Build history of the part. All positions in model axes, mm. Face numbers are marked on the shaded views. A direction names the side the tool comes from. Give positions to 0.01 mm unless a question says otherwise; leave off trailing zeros. Order: outer loops, then holes, each group sorted by start corner. A loop starts at its lowest first (then second) coordinate and runs counter-clockwise, first axis right, second up. Notation, with made-up numbers: (5.25, 19) - (29.25, 19) arc R12 cw to (29.25, 42) - close; hole circle Ø6 at (-14, -32). An arc over 180 degrees is marked (long way). Answer in a Markdown table with one row per item.
```python
from build123d import *

# Parameters (mm, degrees)
SKETCH3_R           = 9.525
SKETCH3_R_2         = 3.175
BOSS_EXTRUDE1_DEPTH = 1.905
SKETCH4_R           = 3.175
BOSS_EXTRUDE2_DEPTH = 4.445


with BuildPart() as part:
    # Sketch3 → Boss-Extrude1 (new body)
    with BuildSketch(Plane(origin=(0, 0, 0), x_dir=(1, 0, 0), z_dir=(0, 1, 0))):
        Circle(SKETCH3_R)
        Circle(SKETCH3_R_2, mode=Mode.SUBTRACT)
    extrude(amount=BOSS_EXTRUDE1_DEPTH)

    # Sketch4 → Boss-Extrude2 (add)
    with BuildSketch(Plane(origin=(0, 1.905, 0), x_dir=(1, 0, 0), z_dir=(0, 1, 0))):
        Polygon((6.647647659, 0), (3.323823829, 5.757031748), (-3.323823829, 5.757031748), (-6.647647659, 0), (-3.323823829, -5.757031748), (3.323823829, -5.757031748), align=None)
        Circle(SKETCH4_R, mode=Mode.SUBTRACT)
    extrude(amount=BOSS_EXTRUDE2_DEPTH)


solid = part.part
```
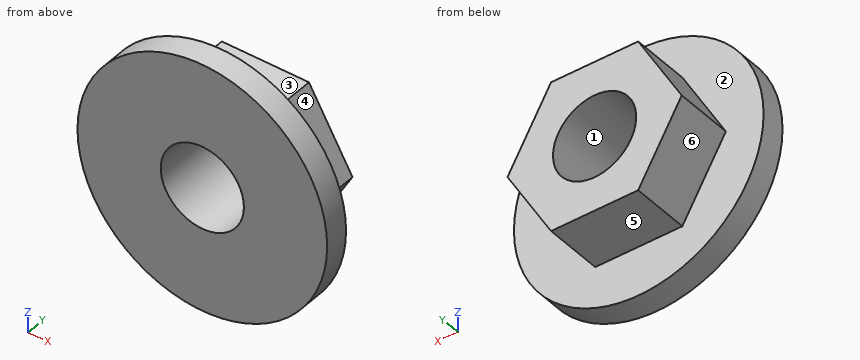
1. Drop flat-ended pins along their axis: P1, Ø1.3, axis at x = -1.5, y = 4, coming from the -Z side; P2, Ø1.3, axis at x = 1, y = 4.5, coming from the +Z side; P3, Ø2, axis at y = 1.5, z = -7.5, coming from the -X side; P4, Ø9.5, axis at x = -0.5, z = 2, coming from the +Y side. Give the stop position or say it passes through.
Check result:
| item | result |
|---|---|
| P1 | stops at z = -5.76 |
| P2 | stops at z = 5.76 |
| P3 | stops at x = -6.96 |
| P4 | stops at y = 6.35 |
2. Cut at D-D on z = -3.5. Write the cut outline in (x, y) (3 decimals).
Check result:
| item | result |
|---|---|
| outline | (-8.859, 0) - (8.859, 0) - (8.859, 1.905) - (4.627, 1.905) - (4.627, 6.35) - (-4.627, 6.35) - (-4.627, 1.905) - (-8.859, 1.905) - close |
3. Which spindle directions (+Z, -Z, +X, -X, +Y, -Y) get a long thin tool onto all of the face, cutting with end or side? Do the marked faces 4, 5 and 6. Say none if no direction does.
Check result:
| item | result |
|---|---|
| face 4 | +Z, +X, +Y |
| face 5 | -Z, +X, -X, +Y |
| face 6 | -Z, -X, +Y |
4. Cut at C-C on x = 6.25. Write the cut outline in (y, z) (3 decimals), and give its area (3 significant figures).
Check result:
| item | result |
|---|---|
| outline | (0, -7.188) - (1.905, -7.188) - (1.905, -0.689) - (6.35, -0.689) - (6.35, 0.689) - (1.905, 0.689) - (1.905, 7.188) - (0, 7.188) - close |
| area | 33.5 mm² |
5. Two-plate mould, pull along Z, no slides. Class the marked faces 1, 2 and 3: +Z half, -Z half, draft (parallel to the pull), parting line (faces both ways), or undercut.
Check result:
| item | result |
|---|---|
| face 1 | undercut |
| face 2 | draft |
| face 3 | +Z half |
6. Cut at B-B on z = 2.75. Write the cut outline in (x, y) (3 decimals), and give its area (3 significant figures).
Check result:
| item | result |
|---|---|
| outline | (-9.119, 0) - (-1.587, 0) - (-1.587, 6.35) - (-5.06, 6.35) - (-5.06, 1.905) - (-9.119, 1.905) - close; (1.587, 0) - (9.119, 0) - (9.119, 1.905) - (5.06, 1.905) - (5.06, 6.35) - (1.587, 6.35) - close |
| area | 59.6 mm² |
7. Cut at A-A on x = 0. Write the cut outline in (y, z) (3 decimals), and give its area (3 significant figures).
Check result:
| item | result |
|---|---|
| outline | (0, -9.525) - (1.905, -9.525) - (1.905, -5.757) - (6.35, -5.757) - (6.35, -3.175) - (0, -3.175) - close; (0, 3.175) - (6.35, 3.175) - (6.35, 5.757) - (1.905, 5.757) - (1.905, 9.525) - (0, 9.525) - close |
| area | 47.1 mm² |
8. Probe line 1 (Z direction, x = 0, y = 3) (3 decimals); line 2 (Y direction, x = 7.75, z = 2.75) (3 decimals); line 3 (Z direction, x = 1.5, y = 1). List the from-to ranges inside material, lowest first.
Check result:
| item | result |
|---|---|
| line 1 | z = -5.757 to -3.175, 3.175 to 5.757 |
| line 2 | y = 0 to 1.905 |
| line 3 | z = -9.41 to -2.8, 2.8 to 9.41 |
